Could you check a few things on this model? Use its own coordinates, in mm. Give positions to 0.01 mm unless a question says otherwise; leave off trailing zeros. One line per item, written item: value.
```python
from build123d import *


# Read off the part's stored shape, not the designer's step: Shell1
with BuildPart() as part:
    # Sketch2 → Revolve1 (revolve)
    with BuildSketch(Plane.XY):
        with BuildLine():
            Line((0, 114.791792001), (-36.226923197, 114.791792001))
            Line((-36.226923197, 114.791792001), (-24.070455057, 88.047562095))
            ThreePointArc((-24.070455057, 88.047562095), (-42.977139074, 0.063432784), (-26.501748685, -88.408207999))
            Line((-26.501748685, -88.408207999), (0, -88.408207999))
            Line((0, -88.408207999), (0, 114.791792001))
        make_face()
    revolve(axis=Axis((0, 114.791792001, 0), (0, -1, 0)))

    # Shell1 outline → Shell1 (revolve, cut)
    with BuildSketch(Plane.XY):
        with BuildLine():
            Line((21.28958956, 88.067845354), (33.436838036, 114.791792001))
            Line((33.436838036, 114.791792001), (0, 114.791792001))
            Line((0, 114.791792001), (0, -85.868207999))
            Line((0, -85.868207999), (24.777861268, -85.868207999))
            ThreePointArc((24.777861268, -85.868207999), (40.413359906, 1.448365664), (21.28958956, 88.067845354))
        make_face()
    revolve(axis=Axis((0, 0, 0), (0, 1, 0)), mode=Mode.SUBTRACT)


solid = part.part
```
1) We'd pull the mould along Z, two halves only. Please class faces 1 (the face through (0, -88.408, 0)), 2 (the face through (0, -85.868, 0)), 3 (the face through (5.346, 89.346, 24.074)), 4 (the face through (-5.072, 92.709, 22.843)): pulls with the +Z half, pulls with the -Z half, needs draft (parallel to the pull), parting line crosses it, or undercut.
Outcome:
face 1: needs draft
face 2: undercut
face 3: parting line crosses it
face 4: undercut
2) I'm going to push flat-ended pins straight in: pin 1 (4 mm diameter, centred on x = -18, z = 23.5, fed in from +Y); pin 2 (10 mm diameter, centred on x = 9, z = 23, fed in from +Y); pin 3 (2 mm diameter, centred on x = -33, z = 31.5, fed in from -Y); pin 4 (5 mm diameter, centred on x = -21, z = -17, fed in from +Y). Where does each tip first touch, or does it pass through?
Outcome:
pin 1: stops at y = 110.75
pin 2: stops at y = 106.57
pin 3: passes through
pin 4: stops at y = 106.17
3) Please list where these lines run through material, in increasing order: L1, parallel to Y at x = -11.5, z = -4; L2, parallel to X at y = -77, z = 9; L3, parallel to X at y = -14.5, z = -34. Write a range as from..to.
Outcome:
L1: y = -88.41..-85.87
L2: x = -29.39..-26.57, 26.57..29.39
L3: x = -25.86..-21.39, 21.39..25.86
